```python
from build123d import *

# Parameters (mm, degrees)
F0_R     = 15
F1_DEPTH = 5
F2_R     = 12.5
F3_DEPTH = 50
F4_R     = 11.75
F5_DEPTH = 1.5
F7_R     = 12.5
F8_DEPTH = 5
F9_SIZE  = 1


with BuildPart() as f1:
    # F0 (on Front) → F1 (new body)
    with BuildSketch(Plane.XZ):
        Circle(F0_R)
    extrude(amount=F1_DEPTH)

    # F2 (on face) → F3 (join)
    with BuildSketch(Plane.XZ.offset(5)):
        Circle(F2_R)
    extrude(amount=F3_DEPTH)

    # F4 (on face) → F5 (join)
    with BuildSketch(Plane.XZ.offset(55)):
        Circle(F4_R)
    extrude(amount=F5_DEPTH)

    # F7 (on face) → F8 (join)
    with BuildSketch(Plane.XZ.offset(56.5)):
        Circle(F7_R)
    extrude(amount=F8_DEPTH)

    # F9
    f9_edges = [f1.edges().sort_by_distance(p)[0] for p in [
        (-12.5, -61.5, 0),
    ]]
    chamfer(f9_edges, length=F9_SIZE)


solid = f1.part
```
Input: part model. Units: mm. Frame: model coordinates. A direction names the side the tool comes from. Round coordinates to 2 decimals unless told otherwise and drop trailing zeros. Loops run counter-clockwise (first coordinate to the right, second up) from the corner with the lowest first, then second, coordinate; pieces in that order, holes last. Notation, with made-up numbers: (34.25, 65.25) -> (69.25, 65.25) arc R10 ccw to (69.25, 72.25) -> close; hole circle Ø9 at (18.25, -1.5). An arc over 180 degrees is marked (long way). Write each question's results on one line, items separated by ' | '.
1. Section B-B (x = 0). Return loops of the section in (y, z), and give its area (3 significant figures).
Geometry results:
outline: (-61.5, -11.5) -> (-60.5, -12.5) -> (-56.5, -12.5) -> (-56.5, -11.75) -> (-55, -11.75) -> (-55, -12.5) -> (-5, -12.5) -> (-5, -15) -> (0, -15) -> (0, 15) -> (-5, 15) -> (-5, 12.5) -> (-55, 12.5) -> (-55, 11.75) -> (-56.5, 11.75) -> (-56.5, 12.5) -> (-60.5, 12.5) -> (-61.5, 11.5) -> close | area: 1,560 mm2
2. First-contact query: P1, Ø4, axis at x = -10, y = -51.5, coming from the -Z side; P2, Ø8, axis at x = -2, y = -28.5, coming from the +Z side; P3, Ø3, axis at x = 4.5, z = -5.5, coming from the +Y side; P4, Ø4, axis at y = -18.5, z = 8, coming from the -X side. Flat tips, straight axial feed; report the tip coordinate or a pass-through.
Geometry results:
P1: z = -9.6 | P2: z = 12.5 | P3: y = 0 | P4: x = -10.97
3. Section C-C (y = -31.5). Return loops of the section in (x, z), and give its area (3 significant figures).
Geometry results:
outline: circle Ø25 at (0, 0) | area: 491 mm2
4. Section A-A (z = 0). Return loops of the section in (x, y).
Geometry results:
outline: (-15, -5) -> (-12.5, -5) -> (-12.5, -55) -> (-11.75, -55) -> (-11.75, -56.5) -> (-12.5, -56.5) -> (-12.5, -60.5) -> (-11.5, -61.5) -> (11.5, -61.5) -> (12.5, -60.5) -> (12.5, -56.5) -> (11.75, -56.5) -> (11.75, -55) -> (12.5, -55) -> (12.5, -5) -> (15, -5) -> (15, 0) -> (-15, 0) -> close
5. Ray query, line 1 (Y direction, x = 3.5, z = 11.25); line 2 (Y direction, x = -9, z = -9.75); line 3 (Y direction, x = 2.25, z = -11.75). Return the intervals inside material, ascending. Write a range as from..to.
Geometry results:
line 1: -61.22..-56.5, -55..0 | line 2: -5..0 | line 3: -61.04..-56.5, -55..0
6. Mould query, pull axis Y, two halves, no side actions, for faces 1 (the face through (11, -56.5, -5)), 2 (the face through (-14.985, -2.465, 0.66)), 3 (the face through (0, -61.5, 0)), 4 (the face through (0, 0, 0)). Classes: +Y half, -Y half, draft (parallel to the pull), parting line (faces both ways), or undercut.
Geometry results:
face 1: undercut | face 2: draft | face 3: -Y half | face 4: +Y half
7. Set-up query: faces 5 (the face through (-3.4, -5, 12.3)), 6 (the face through (11, -55, -5)). Return all of +Z, -Z, +X, -X, +Y, -Y with unobstructed straight access to the full face (end or side cutting, diameter ignored); none if empty.
Geometry results:
face 5: -Y | face 6: none
